Can you work these out from the model? Positions are in its coordinate system, mm. A direction names the side the tool comes from. Give positions to 0.01 mm unless a question says otherwise; leave off trailing zeros. Answer as CSV lines item,"result".
```python
from build123d import *

# Parameters (mm, degrees)
DOME2_FACE_RADIUS               = 3.1
DOME2_HEIGHT                    = 0.8
SKETCH6_R                       = 0.500000006
CUT_EXTRUDE2_DEPTH              = 1
SKETCH7_R                       = 0.75
CUT_EXTRUDE3_DEPTH              = 1
BOSS_EXTRUDE1_REACH             = 12.152
SKETCH9_R                       = 1
SKETCH9_R_2                     = 0.45
BOSS_EXTRUDE1_DIRECTION_2_DEPTH = 0.5


with BuildPart() as part:
    # Sketch2 → Revolve2 (revolve)
    with BuildSketch(Plane.XY):
        with BuildLine():
            Line((0, 0), (3.1, 0))
            add(Edge.make_bspline(
                [(0, -10.151978408), (2.177642547, -9.857333884), (3.515065362, -5.793498011), (3.1, 0)],
                knots=[0, 0, 0, 0, 1, 1, 1, 1], degree=3))
            Line((0, -10.151978408), (0, 0))
        make_face()
    revolve(axis=Axis((0, -10.151978408, 0), (0, 1, 0)))

    # Dome2: a dome of height H over a round flat face of radius A is a cap of a sphere of radius (A * A + H * H) / (2 * H)
    dome2_r = (DOME2_FACE_RADIUS * DOME2_FACE_RADIUS + DOME2_HEIGHT * DOME2_HEIGHT) / (2 * DOME2_HEIGHT)
    dome2_base = Plane((0, 0, 0), z_dir=(0, -1, 0))
    with Locations(dome2_base.offset(DOME2_HEIGHT - dome2_r)):
        dome2_ball = Sphere(dome2_r, mode=Mode.PRIVATE)
    add(split(dome2_ball, bisect_by=dome2_base, keep=Keep.TOP, mode=Mode.PRIVATE), mode=Mode.SUBTRACT)

    # Sketch6 → Cut-Extrude2 (cut, symmetric)
    with BuildSketch(Plane(origin=(3.16696636, 0, 0), x_dir=(0, 0, -1), z_dir=(1, 0, 0))):
        with Locations((0, -1.377313707)):
            Circle(SKETCH6_R)
    cut_extrude2 = extrude(amount=CUT_EXTRUDE2_DEPTH, both=True, mode=Mode.SUBTRACT)

    # Mirror1: Cut-Extrude2 across plane
    add(cut_extrude2.mirror(Plane(origin=(0, 0, 0), x_dir=(0, 0, 1), z_dir=(1, 0, 0))), mode=Mode.SUBTRACT)

    # Sketch7 → Cut-Extrude3 (cut)
    with BuildSketch(Plane(origin=(0, 0, 0), x_dir=(1, 0, 0), z_dir=(0, 1, 0))):
        Circle(SKETCH7_R)
    extrude(amount=-CUT_EXTRUDE3_DEPTH, mode=Mode.SUBTRACT)

    # Sketch9 → Boss-Extrude1 (add, up to next)
    with BuildSketch(Plane(origin=(0, -10.151978408, 0), x_dir=(1, 0, 0), z_dir=(0, 1, 0)), mode=Mode.PRIVATE) as boss_extrude1_sk1:
        Circle(SKETCH9_R)
        Circle(SKETCH9_R_2, mode=Mode.SUBTRACT)
    boss_extrude1_tool1 = extrude(boss_extrude1_sk1.sketch, amount=BOSS_EXTRUDE1_REACH, mode=Mode.PRIVATE) - part.part
    add(boss_extrude1_tool1.solids().sort_by_distance((-0.971716, -10.151978, 0))[0])

    # Sketch9 → Boss-Extrude1 direction 2 (add)
    with BuildSketch(Plane(origin=(0, -10.151978408, 0), x_dir=(1, 0, 0), z_dir=(0, 1, 0))):
        Circle(SKETCH9_R)
        Circle(SKETCH9_R_2, mode=Mode.SUBTRACT)
    extrude(amount=-BOSS_EXTRUDE1_DIRECTION_2_DEPTH)


solid = part.part
```
Item 1: We'd pull the mould along Y, two halves only. Please class faces 1 (the cylindrical face through (-2.678, -0.882, 0.065)), 2 (the flat face through (0, -1, 0)): released by +Y, released by -Y, zero draft, split by the parting line, or undercut.
Numbers:
face 1,"undercut"
face 2,"released by +Y"
Item 2: For faces 3 (the flat face through (-2.167, -1.4, 0)), 4 (the cylindrical face through (2.678, -0.882, 0.065)), which set-ups out of +Z, -Z, +X, -X, +Y, -Y let a thin tool reach every point of the face, with its end or its side?
Numbers:
face 3,"-X"
face 4,"+X"
Item 3: For pin 1 (1 mm diameter, centred on y = -1.5, z = 1, fed in from -X); pin 2 (1.6 mm diameter, centred on x = 0.5, z = 0, fed in from +Y); pin 3 (0.5 mm diameter, centred on y = -1.5, z = 0, fed in from +X), each with a flat end and sliding along its axis, tell me the tip position at first contact or that it passes through.
Numbers:
pin 1,"stops at x = -3.13"
pin 2,"stops at y = -0.67"
pin 3,"stops at x = 2.17"
Item 4: Please list where these lines run through material, in increasing order: line 1 along X through (y, z) = (-10.35, 0); line 2 along Z through (x, y) = (-2.25, -1); line 3 along Y through (x, z) = (0.5, -1).
Numbers:
line 1,"x = -1 to -0.45, 0.45 to 1"
line 2,"z = -2.21 to -0.33, 0.33 to 2.21"
line 3,"y = -9.61 to -0.7"
